```python
from build123d import *

# Parameters (mm, degrees)
SKETCH1_R               = 34.555
BOSS_EXTRUDE1_DEPTH     = 12.75
SKETCH2_R               = 3.35
CUT_EXTRUDE1_DEPTH      = 51.504044888
CIRPATTERN1_COUNT       = 6
SKETCH6_R               = 24.23
CUT_EXTRUDE3_DEPTH      = 1
CUT_EXTRUDE2_DEPTH      = 51.504044888
CUT_EXTRUDE2_DEPTH_BACK = 51.504044888
SKETCH4_R               = 2
CUT_EXTRUDE4_DEPTH      = 52.727217057
CUT_EXTRUDE4_DEPTH_BACK = 52.727217057
SKETCH9_R               = 1


with BuildPart() as part:
    # Sketch1 → Boss-Extrude1 (new body)
    with BuildSketch(Plane(origin=(0, 0, 0), x_dir=(1, 0, 0), z_dir=(0, 1, 0))):
        with Locations(Location((0, 0, 0), (0, 0, 270))):
            Circle(SKETCH1_R)
    extrude(amount=BOSS_EXTRUDE1_DEPTH)

    # Sketch2 → Cut-Extrude1 (cut, through all)
    with BuildSketch(Plane(origin=(0, 12.75, 0), x_dir=(1, 0, 0), z_dir=(0, 1, 0))):
        with Locations(Location((0, 29.35, 0), (0, 0, 270))):
            Circle(SKETCH2_R)
    cut_extrude1 = extrude(amount=-CUT_EXTRUDE1_DEPTH, mode=Mode.SUBTRACT)

    # CirPattern1: Cut-Extrude1 ×6 about axis
    cirpattern1_axis = Axis((0, 0, 0), (0, 1, 0))
    for i in range(1, CIRPATTERN1_COUNT):
        add(cut_extrude1.rotate(cirpattern1_axis, i * 360 / CIRPATTERN1_COUNT), mode=Mode.SUBTRACT)

    # Sketch6 → Cut-Extrude3 (cut)
    with BuildSketch(Plane.XZ):
        with Locations(Location((0, 0, 0), (0, 0, 270))):
            Circle(SKETCH6_R)
    cut_extrude3 = extrude(amount=-CUT_EXTRUDE3_DEPTH, mode=Mode.SUBTRACT)

    # Sketch7 → Revolve1 (revolve)
    with BuildSketch(Plane(origin=(0, 0, 0), x_dir=(0, 0, -1), z_dir=(1, 0, 0))):
        Polygon((24.23, 1), (20.98, 0.5334), (20.98, 1), align=None)
    revolve1 = revolve(axis=Axis((0, 0, 0), (0, 1, 0)))

    # Mirror1: Cut-Extrude3 across plane
    add(cut_extrude3.mirror(Plane(origin=(0, 6.375, 0), x_dir=(0, 0, 1), z_dir=(0, -1, 0))), mode=Mode.SUBTRACT)

    # Mirror2: Revolve1 across plane
    add(revolve1.mirror(Plane(origin=(0, 6.375, 0), x_dir=(0, 0, 1), z_dir=(0, -1, 0))))

    # Sketch4 → Cut-Extrude2 (cut, two sides: drawn at the far end of the back side and taken through both)
    with BuildSketch(Plane(origin=(0, 0, 0), x_dir=(0, 0, -1), z_dir=(1, 0, 0)).offset(-CUT_EXTRUDE2_DEPTH_BACK)):
        with Locations((0, 14.25)):
            Circle(SKETCH4_R)
        with Locations((0, -1.5)):
            Circle(SKETCH4_R)
    extrude(amount=CUT_EXTRUDE2_DEPTH + CUT_EXTRUDE2_DEPTH_BACK, mode=Mode.SUBTRACT)

    # Sketch9 → Cut-Extrude4 (cut, two sides: drawn at the far end of the back side and taken through both)
    with BuildSketch(Plane(origin=(0, 0.710347248, 2.005958746), x_dir=(1, 0, 0), z_dir=(0, 0.33380685923377496, 0.942641491092177)).offset(-CUT_EXTRUDE4_DEPTH_BACK)):
        with Locations(Location((0, 6.009339506, 0), (0, 0, 270))):
            Circle(SKETCH9_R)
    extrude(amount=CUT_EXTRUDE4_DEPTH + CUT_EXTRUDE4_DEPTH_BACK, mode=Mode.SUBTRACT)


solid = part.part
```
Build history of the part. All positions in model axes, mm. A direction names the side the tool comes from. Coordinates: 2 decimals unless noted, no trailing zeros. Order: outer loops, then holes, each group sorted by start corner. A loop starts at its lowest first (then second) coordinate and runs counter-clockwise, first axis right, second up.
Item 1: Mould opens along X. For faces 4 (the cylindrical face through (-22.148, 6.464, -13.949)), 5 (the cylindrical face through (-21.03, 6.29, -27.42)), 6 (the cylindrical face through (-0.383, 5.396, 0.003)), 7 (the flat face through (0, 12.75, 25)) say: released by +X, released by -X, zero draft, split by the parting line, or undercut.
Filled in:
face 4: undercut
face 5: split by the parting line
face 6: undercut
face 7: zero draft
Item 2: Drill centre lines: L1, parallel to Z at x = -23, y = 5.25; L2, parallel to X at y = 5.5, z = 14; L3, parallel to Z at x = -27, y = 10.5. Where is each one in solid material? Low to high.
Filled in:
L1: z = -25.79 to -16.99, -12.36 to 12.36, 16.99 to 25.79
L2: x = -31.59 to -28.7, -22.14 to 22.14, 28.7 to 31.59
L3: z = -21.56 to -17.63, -11.72 to 11.72, 17.63 to 21.56
Item 3: Tool access for faces 1 (the cylindrical face through (-29.45, 12.25, 0.02)), 2 (the flat face through (0, 11.75, 0)), 3 (the cylindrical face through (12.766, 0.77, 16.649)): list every direction of +Z, -Z, +X, -X, +Y, -Y with a clear straight run to the whole face (end or side of a thin tool).
Filled in:
face 1: +X, -X, +Y
face 2: +Y
face 3: -Y
Item 4: Drop flat-ended pins along their axis: pin 1 Ø5 at (x, y) = (-10, 8) entering from +Z; pin 2 Ø21 at (x, z) = (-8, 8.5) entering from +Y; pin 3 Ø2 at (x, y) = (25.5, 10) entering from -Z; pin 4 Ø4 at (x, z) = (-25.42, -14.68) entering from +Y. Give the stop position or say it passes through.
Filled in:
pin 1: stops at z = 33.73
pin 2: stops at y = 12.22
pin 3: stops at z = -24.37
pin 4: passes through
Item 5: Saw through at A-A on z = -29.35. List the corners of the cut face in (x, y).
Filled in:
outline: (-18.24, 0) - (-3.35, 0) - (-3.35, 12.75) - (-18.24, 12.75) - close; (3.35, 0) - (18.24, 0) - (18.24, 12.75) - (3.35, 12.75) - close
Item 6: Saw through at B-B on x = 0. State how many separate pieces and enclosed holes the cut face has, then the cut area to 3 significant figures.
Filled in:
separate pieces: 4
enclosed holes: 0
area: 552 mm2
